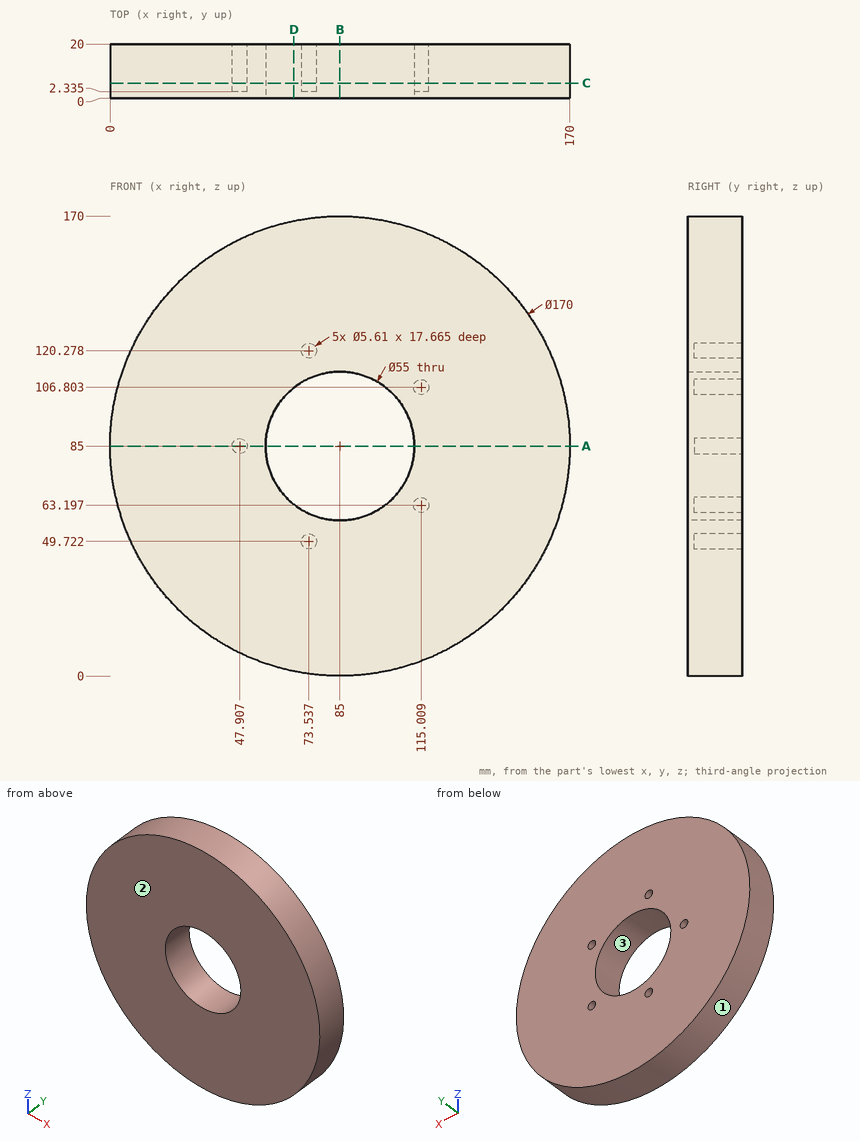
The drawing under review shows one solid part. Ordinate dimensions are in mm from its lowest x, y, z. Give positions to 0.01 mm unless a question says otherwise; leave off trailing zeros. Loops run counter-clockwise (first coordinate to the right, second up) from the corner with the lowest first, then second, coordinate; pieces in that order, holes last. Notation, with made-up numbers: M 38,81.25 L 95,81.25 A15 ccw 95,106.25 Z; hole C 22.5,84 d10. An arc over 180 degrees is marked long. Return JSON: item names as keys, results as strings. Group by question number.
Item 1: We need section B-B (x = 85). Give the boundary of the cut face in (y, z), and give its area (3 significant figures).
Item 2: We need section C-C (y = 5.5). Give the boundary of the cut face in (x, z) (1 decimal), and give its area (3 significant figures).
Item 3: Insertion check: pin 1 Ø4.5 at (x, z) = (115, 63.5) entering from +Y (1 decimal); pin 2 Ø3 at (y, z) = (3.5, 62.5) entering from -X (1 decimal); pin 3 Ø4 at (x, y) = (115, 4) entering from -Z (1 decimal). Each pin has a flat end and moves straight along its axis. Give the tip position at first contact, or say it passes through.
Item 4: We need section D-D (x = 68). Give the boundary of the cut face in (y, z) (1 decimal), and give its area (3 significant figures).
Item 5: We need section A-A (z = 85). Give the boundary of the cut face in (x, y) (1 decimal), and give its area (3 significant figures).
Item 6: For probe 1 along X at (y, z) = (7.25, 85); probe 2 along Z at (x, y) = (113.5, 3) (1 decimal); probe 3 along Z at (x, y) = (76, 1.5) (1 decimal), list the stretches that pass through material, from the lowest coordinate up.
Item 7: Mouldability with a two-part tool opening along X and no side actions: class the marked faces 1, 2 and 3 as released by +X, released by -X, zero draft, split by the parting line, or undercut.
Output:
{
 "1": {"outline": "M 0,0 L 20,0 L 20,57.5 L 0,57.5 Z; M 0,112.5 L 20,112.5 L 20,170 L 0,170 Z", "area": "2,300 mm^2"},
 "2": {"outline": "C 85,85 d170; hole C 47.9,85 d5.6; hole C 85,85 d55; hole C 73.5,49.7 d5.6; hole C 73.5,120.3 d5.6; hole C 115,63.2 d5.6; hole C 115,106.8 d5.6", "area": "20,200 mm^2"},
 "3": {"pin 1": "stops at y = 2.3", "pin 2": "stops at x = 2.6", "pin 3": "stops at z = 4.7"},
 "4": {"outline": "M 0,1.7 L 20,1.7 L 20,63.4 L 0,63.4 Z; M 0,106.6 L 20,106.6 L 20,168.3 L 0,168.3 Z", "area": "2,470 mm^2"},
 "5": {"outline": "M 0,0 L 57.5,0 L 57.5,20 L 50.7,20 L 50.7,2.3 L 45.1,2.3 L 45.1,20 L 0,20 Z; M 112.5,0 L 170,0 L 170,20 L 112.5,20 Z", "area": "2,200 mm^2"},
 "6": {"probe 1": "x = 0 to 45.1, 50.71 to 57.5, 112.5 to 170", "probe 2": "z = 4.9 to 60.8, 65.6 to 104.4, 109.2 to 165.1", "probe 3": "z = 0.5 to 59, 111 to 169.5"},
 "7": {"face 1": "split by the parting line", "face 2": "zero draft", "face 3": "undercut"}
}
